Can you work these out from the model? Positions are in its coordinate system, mm. Face numbers are marked on the shaded views. A direction names the side the tool comes from. Round coordinates to 2 decimals unless told otherwise and drop trailing zeros. Order: outer loops, then holes, each group sorted by start corner. A loop starts at its lowest first (then second) coordinate and runs counter-clockwise, first axis right, second up. Notation, with made-up numbers: M -11.5,86 L 23.5,86 A20 cw 23.5,120 Z; hole C -35,89.5 d2. An arc over 180 degrees is marked long. One line per question, with ' | ' between items.
Autodesk Fusion 360 part; units mm, degrees
sketch "Sketch1" plane through (0, 0, 0) normal (0, 0, 1) x (1, 0, 0)
  line L0 (1, 0) -> (18, 0)
  line L1 (19, 1) -> (19, 18)
  line L2 (18, 19) -> (1, 19)
  line L3 (0, 18) -> (0, 1)
  arc A0 (1, 19) -> (0, 18) centre (1, 18) ccw
  arc A1 (19, 18) -> (18, 19) centre (18, 18) ccw
  arc A2 (18, 0) -> (19, 1) centre (18, 1) ccw
  arc A3 (0, 1) -> (1, 0) centre (1, 1) ccw
  line L4 (18.7071, 18.7071) -> (0.2929, 0.2929) construction
  line L5 (18.7071, 0.2929) -> (0.2929, 18.7071) construction
  line L6 (2, 17) -> (17, 17)
  line L7 (17, 17) -> (17, 2)
  line L8 (17, 2) -> (2, 2)
  line L9 (2, 2) -> (2, 17)
  line L10 (17, 17) -> (2, 2) construction
  line L11 (2, 17) -> (17, 2) construction
  point P0 (19, 0)
  point P1 (0, 19)
  point P2 (9.5, 9.5)
  point P3 (9.5, 9.5)
  dimension "d1" = 19
  dimension "d2" = 19
  dimension "d3" = 1
  dimension "d4" = 1
  dimension "d5" = 1
  dimension "d6" = 1
  dimension "d7" = 15
  dimension "d8" = 15
extrude "Extrude1" add sketch "Sketch1" along normal blind 3 makes body 1
sketch "Sketch2" plane through (0, 0, 3) normal (0, 0, 1) x (-1, 0, 0)
  line L0 (-17, -2) -> (-2, -2)
  line L1 (-2, -2) -> (-2, -17)
  line L2 (-2, -17) -> (-17, -17)
  line L3 (-17, -17) -> (-17, -2)
  arc A0 (0, -1) -> (-1, 0) centre (-1, -1) ccw
  line L4 (-1, 0) -> (-18, 0)
  arc A1 (-18, 0) -> (-19, -1) centre (-18, -1) ccw
  line L5 (-19, -1) -> (-19, -18)
  arc A2 (-19, -18) -> (-18, -19) centre (-18, -18) ccw
  line L6 (-18, -19) -> (-1, -19)
  arc A3 (-1, -19) -> (0, -18) centre (-1, -18) ccw
  line L7 (0, -18) -> (0, -1)
  line L8 (-17, -2) -> (-2, -17) construction
  line L9 (-2, -2) -> (-17, -17) construction
  line L10 (-9.5, -9.5) -> (-17, -9.5) construction
  line L11 (-9.5, -9.5) -> (-2, -9.5) construction
  line L12 (-17, -11.5) -> (-2, -11.5)
  line L13 (-17, -7.5) -> (-2, -7.5)
  line L14 (-2, -7.5) -> (-2, -11.5)
  line L15 (-17, -11.5) -> (-17, -7.5)
  line L16 (-7.75, -10.75) -> (-11.25, -10.75)
  line L17 (-11.25, -10.75) -> (-11.25, -8.25)
  line L18 (-11.25, -8.25) -> (-7.75, -8.25)
  line L19 (-7.75, -8.25) -> (-7.75, -10.75)
  line L20 (-11.25, -8.25) -> (-7.75, -10.75) construction
  line L21 (-11.25, -10.75) -> (-7.75, -8.25) construction
  point P0 (-9.5, -9.5)
  point P1 (-9.5, -9.5)
  dimension "d11" = 2
  dimension "d12" = 2
  dimension "d13" = 3.5
  dimension "d14" = 2.5
extrude "Extrude2" add sketch "Sketch2" along normal blind 4 separate body contours L1 L3 L12 L13 L14 L15 makes body 2
extrude "Extrude3" add 1 faces at (0.6667, 7, 3) along direction (0, 0, 1) blind 4 on bodies 1 bodies 1 2
sketch "Sketch3" plane through (0, 11.5, 0) normal (0, 1, 0) x (-1, 0, 0)
  line L0 (-17, 3) -> (-2, 3)
  line L1 (-2, 3) -> (-2, 7)
  line L2 (-2, 7) -> (-17, 7)
  line L3 (-17, 7) -> (-17, 3)
sketch "Sketch4" plane through (0, 0, 7) normal (0, 0, 1) x (-1, 0, 0)
  line L0 (-17, -7.5) -> (-17, -2)
  line L1 (-17, -2) -> (-2, -2)
  line L2 (-2, -2) -> (-2, -7.5)
  line L3 (-2, -7.5) -> (-17, -7.5)
  line L4 (-11.25, -8.25) -> (-7.75, -8.25)
  line L5 (-7.75, -8.25) -> (-7.75, -10.75)
  line L6 (-7.75, -10.75) -> (-11.25, -10.75)
  line L7 (-11.25, -10.75) -> (-11.25, -8.25)
  line L8 (-17, -11.5) -> (-2, -11.5)
  line L9 (-2, -11.5) -> (-2, -17)
  line L10 (-2, -17) -> (-17, -17)
  line L11 (-17, -17) -> (-17, -11.5)
  arc A0 (0, -1) -> (-1, 0) centre (-1, -1) ccw
  line L12 (-1, 0) -> (-18, 0)
  arc A1 (-18, 0) -> (-19, -1) centre (-18, -1) ccw
  line L13 (-19, -1) -> (-19, -18)
  arc A2 (-19, -18) -> (-18, -19) centre (-18, -18) ccw
  line L14 (-18, -19) -> (-1, -19)
  arc A3 (-1, -19) -> (0, -18) centre (-1, -18) ccw
  line L15 (0, -18) -> (0, -1)
  line L16 (-17, -11.5) -> (-2, -17) construction
  line L17 (-2, -11.5) -> (-17, -17) construction
  line L18 (-17, -2) -> (-2, -7.5) construction
  line L19 (-2, -2) -> (-17, -7.5) construction
  line L20 (-17, -11.5) -> (-2, -11.5)
  line L21 (-2, -11.5) -> (-17, -17) construction
  line L22 (-2, -17) -> (-17, -17)
  circle A4 centre (-9.5, -14.25) radius 1.8
  line L23 (-2, -11.5) -> (-2, -17)
  line L24 (-17, -11.5) -> (-2, -17) construction
  line L25 (-17, -17) -> (-17, -11.5)
  line L26 (-2, -7.5) -> (-17, -7.5)
  circle A5 centre (-9.5, -4.75) radius 1.8
  line L27 (-2, -2) -> (-2, -7.5)
  line L28 (-2, -2) -> (-17, -7.5) construction
  line L29 (-17, -7.5) -> (-17, -2)
  line L30 (-17, -2) -> (-2, -2)
  line L31 (-17, -2) -> (-2, -7.5) construction
  point P0 (-9.5, -14.25)
  point P1 (-9.5, -4.75)
  point P2 (-9.5, -14.25)
  point P3 (-9.5, -4.75)
  dimension "d22" = 15
  dimension "d23" = 5.5
  dimension "d24" = 3.6
  dimension "d25" = 15
  dimension "d26" = 5.5
  dimension "d27" = 3.6
extrude "Extrude4" add sketch "Sketch4" along normal blind 2 separate body contours L0 L1 L2 L3 L26 L27 L29 L30 | L8 L9 L10 L11 L20 L22 L23 L25 makes body 3 at (3.9, 14.25, 7) makes body 4 at (15.1, 4.75, 7)
extrude "Extrude5" add 1 faces at (15.0833, 9.9167, 7) along direction (0, 0, 1) blind 2 on bodies 1 bodies 1 3 4
sketch "Sketch5" plane through (19, 0, 0) normal (1, 0, 0) x (0, 1, 0)
  line L0 (1, 0) -> (18, 0)
  line L1 (18, 0) -> (18, 9)
  line L2 (18, 9) -> (1, 9)
  line L3 (1, 9) -> (1, 0)
  line L4 (18, 0) -> (18, 4) construction
  line L5 (18, 4) -> (1, 4)
  line L6 (1, 4) -> (1, 7)
  line L7 (1, 7) -> (18, 7)
  line L8 (18, 7) -> (18, 4)
  dimension "d32" = 4
  dimension "d33" = 3
extrude "Extrude6" add sketch "Sketch5" along normal blind 3 contours L1 L3 L5 L6 L7 L8 bodies 1
sketch "Sketch6" plane through (0, 0, 0) normal (-1, 0, 0) x (0, -1, 0)
  line L0 (-18, 0) -> (-1, 0)
  line L1 (-1, 0) -> (-1, 9)
  line L2 (-1, 9) -> (-18, 9)
  line L3 (-18, 9) -> (-18, 0)
  line L4 (-1, 0) -> (-1, 4) construction
  line L5 (-1, 4) -> (-18, 4)
  line L6 (-18, 4) -> (-18, 7)
  line L7 (-18, 7) -> (-1, 7)
  line L8 (-1, 7) -> (-1, 4)
  dimension "d36" = 4
  dimension "d37" = 3
extrude "Extrude7" add sketch "Sketch6" along normal blind 3 contours L1 L3 L5 L6 L7 L8 bodies 1
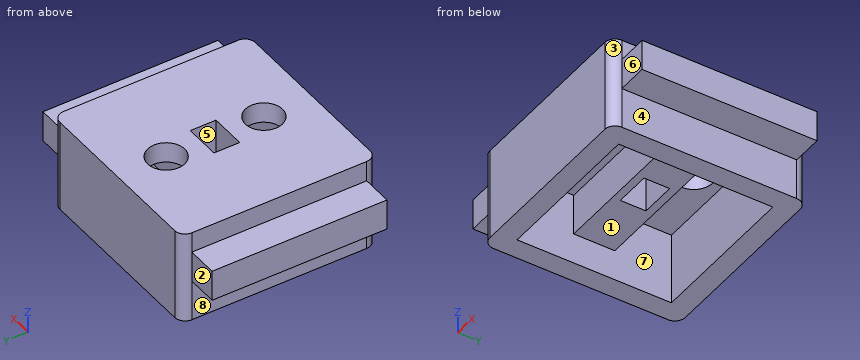
(1) Please list where these lines run through material, in increasing order: probe 1 along Y at (x, z) = (7, 4.5); probe 2 along Y at (x, z) = (9.5, 8.1); probe 3 along X at (y, z) = (4.75, 8). Write a range as [from, to].
Final values:
probe 1: [0, 2], [7.5, 11.5], [17, 19] | probe 2: [0, 2.95], [6.55, 8.25], [10.75, 12.45], [16.05, 19] | probe 3: [0, 7.7], [11.3, 19]
(2) Will these pins go through, and if not, where does the flat tip stop? pin 1 Ø1.6 at (y, z) = (12, 8.5) entering from +X; pin 2 Ø1.5 at (x, z) = (14.5, 3) entering from -Y; pin 3 Ø3.5 at (x, z) = (-2, 6) entering from -Y; pin 4 Ø2.5 at (x, y) = (-1.5, 12.5) entering from -Z.
Final values:
pin 1: x = 19 | pin 2: y = 0 | pin 3: y = 1 | pin 4: z = 4
(3) If we section it at B-B on y = 4.75: Please give me the cut outline in (x, z), plus the area to 3 significant figures.
Final values:
outline: M -3,4 L 0,4 L 0,0 L 2,0 L 2,7 L 7.7,7 L 7.7,9 L 0,9 L 0,7 L -3,7 Z; M 11.3,7 L 17,7 L 17,0 L 19,0 L 19,4 L 22,4 L 22,7 L 19,7 L 19,9 L 11.3,9 Z | area: 76.8 mm^2
(4) If we section it at C-C on z = 1: Please give me the cut outline in (x, y), plus the area to 3 significant figures.
Final values:
outline: M 0,1 A1 ccw 1,0 L 18,0 A1 ccw 19,1 L 19,18 A1 ccw 18,19 L 1,19 A1 ccw 0,18 Z; hole M 2,2 L 17,2 L 17,17 L 2,17 Z | area: 135 mm^2
(5) If we section it at D-D on y = 16.5: Please give me the cut outline in (x, z), plus the area to 3 significant figures.
Final values:
outline: M -3,4 L 0,4 L 0,0 L 2,0 L 2,7 L 17,7 L 17,0 L 19,0 L 19,4 L 22,4 L 22,7 L 19,7 L 19,9 L 0,9 L 0,7 L -3,7 Z | area: 84.0 mm^2
(6) Thinking about a two-plate mould opening in Y: for the marked faces 1, 2, 3 and 4, which applies, released by +Y, released by -Y, zero draft, split by the parting line, or undercut?
Final values:
face 1: undercut | face 2: released by +Y | face 3: released by -Y | face 4: zero draft
(7) On a 3-axis mill with a long thin cutter (end or side, diameter ignored), from which of +Z, -Z, +X, -X, +Y, -Y can I reach the whole of each face in a straight line? I mean the marked faces 5, 6, 7 and 8. Say none if no direction works.
Final values:
face 5: +Z, -Z | face 6: +Z, -Z, +X, -Y | face 7: -Z | face 8: -Z, -X, +Y, -Y
(8) If we section it at A-A on x = 9.5: Please give me the cut outline in (y, z), plus the area to 3 significant figures.
Final values:
outline: M 0,0 L 2,0 L 2,7 L 2.95,7 L 2.95,9 L 0,9 Z; M 6.55,7 L 7.5,7 L 7.5,3 L 8.25,3 L 8.25,9 L 6.55,9 Z; M 10.75,3 L 11.5,3 L 11.5,7 L 12.45,7 L 12.45,9 L 10.75,9 Z; M 16.05,7 L 17,7 L 17,0 L 19,0 L 19,9 L 16.05,9 Z | area: 52.6 mm^2
